Build history of the part. All positions in model axes, mm. A direction names the side the tool comes from. Give positions to 0.01 mm unless a question says otherwise; leave off trailing zeros. Order: outer loops, then holes, each group sorted by start corner. A loop starts at its lowest first (then second) coordinate and runs counter-clockwise, first axis right, second up. Notation, with made-up numbers: M -19,57.25 L -12,57.25 A31 cw -12,93.25 Z; hole C 28.5,13 d2. An arc over 180 degrees is marked long. Use CSV: the item, a comma, the result in double quotes. Start each with the question number.
Item 1: Band-saw the part on C-C on y = 14.25. Write the cut outline in (x, z).
Item 2: Two-plate mould, pull along X, no slides. Class faces 4 (the flat face through (-14.4, 13, 5.2)), 5 (the cylindrical face through (-4.769, -0.74, -21.477)), 6 (the cylindrical face through (3, 10, 0)): pulls with the +X half, pulls with the -X half, needs draft (parallel to the pull), parting line crosses it, or undercut.
Item 3: Band-saw the part on A-A on x = 0. Write the cut outline in (y, z).
Item 4: Wall check: line 1 along Y through (x, z) = (19.5, -9); line 2 along Z through (x, y) = (0, 11.25); line 3 along Y through (x, z) = (-9.5, -13). Give the ranges that are in metal, low to high.
Item 5: Band-saw the part on D-D on z = -11. Write the cut outline in (x, y).
Item 6: Which spindle directions (+Z, -Z, +X, -X, +Y, -Y) get a long thin tool onto all of the face, cutting with end or side? Do faces 1 (the flat face through (15, 11.5, -15)), 2 (the flat face through (0, -1.5, -5)), 3 (the cylindrical face through (14.985, 16.944, 0.66)). Say none if no direction does.
Item 7: Pin check, flat tips, straight feed: P1, Ø1.5, axis at x = -11.5, y = 10.5, coming from the -Z side; P2, Ø10, axis at y = 12, z = -17.5, coming from the -X side; P3, Ø3, axis at y = 4.5, z = -12, coming from the +X side; P4, Ø5, axis at x = 0, z = 0, coming from the -Y side. Stop position of each tip, or through.
Item 8: Band-saw the part on B-B on z = 0. Write the cut outline in (x, y), plus the area to 3 significant figures.
from build123d import *

# Parameters (mm, degrees)
F0_R     = 22
F1_DEPTH = 1.5
F2_R     = 20.69
F3_DEPTH = 11.5
F4_R     = 22
F5_DEPTH = 1.5
F6_R     = 15
F7_DEPTH = 8
F8_R     = 3
F9_DEPTH = 22.501


with BuildPart() as f1:
    # F0 (on Front) → F1 (new body)
    with BuildSketch(Plane.XZ):
        Circle(F0_R)
    extrude(amount=F1_DEPTH)

    # F2 (on face) → F3 (join)
    with BuildSketch(Plane(origin=(0, 0, 0), x_dir=(-1, 0, 0), z_dir=(0, 1, 0))):
        Circle(F2_R)
    extrude(amount=F3_DEPTH)

    # F4 (on face) → F5 (join)
    with BuildSketch(Plane(origin=(0, 11.5, 0), x_dir=(-1, 0, 0), z_dir=(0, 1, 0))):
        Circle(F4_R)
    extrude(amount=F5_DEPTH)

    # F6 (on face) → F7 (join)
    with BuildSketch(Plane(origin=(0, 13, 0), x_dir=(-1, 0, 0), z_dir=(0, 1, 0))):
        Circle(F6_R)
    extrude(amount=F7_DEPTH)

    # F8 (on face) → F9 (cut, through all)
    with BuildSketch(Plane(origin=(0, 21, 0), x_dir=(-1, 0, 0), z_dir=(0, 1, 0))):
        Circle(F8_R)
    extrude(amount=-F9_DEPTH, mode=Mode.SUBTRACT)


solid = f1.part
Model answer:
1,outline,"C 0,0 d30; hole C 0,0 d6"
2,face 4,"needs draft"
2,face 5,"parting line crosses it"
2,face 6,"undercut"
3,outline,"M -1.5,-22 L 0,-22 L 0,-20.69 L 11.5,-20.69 L 11.5,-22 L 13,-22 L 13,-15 L 21,-15 L 21,-3 L -1.5,-3 Z; M -1.5,3 L 21,3 L 21,15 L 13,15 L 13,22 L 11.5,22 L 11.5,20.69 L 0,20.69 L 0,22 L -1.5,22 Z"
4,line 1,"y = -1.5 to 0, 11.5 to 13"
4,line 2,"z = -20.69 to -3, 3 to 20.69"
4,line 3,"y = -1.5 to 13"
5,outline,"M -19.05,-1.5 L 19.05,-1.5 L 19.05,0 L 17.52,0 L 17.52,11.5 L 19.05,11.5 L 19.05,13 L 10.2,13 L 10.2,21 L -10.2,21 L -10.2,13 L -19.05,13 L -19.05,11.5 L -17.52,11.5 L -17.52,0 L -19.05,0 Z"
6,face 1,"none"
6,face 2,"+Z, -Z, +X, -X, -Y"
6,face 3,"+Y"
7,P1,"stops at z = -17.68"
7,P2,"stops at x = -18.1"
7,P3,"stops at x = 17.83"
7,P4,"passes through"
8,outline,"M -22,-1.5 L -3,-1.5 L -3,21 L -15,21 L -15,13 L -22,13 L -22,11.5 L -20.69,11.5 L -20.69,0 L -22,0 Z; M 3,-1.5 L 22,-1.5 L 22,0 L 20.69,0 L 20.69,11.5 L 22,11.5 L 22,13 L 15,13 L 15,21 L 3,21 Z"
8,area,"713 mm^2"
